The listing builds one solid part. Answer for the finished solid, in the listing's coordinates (mm). A direction names the side the tool comes from. Coordinates: 2 decimals unless noted, no trailing zeros. Loops run counter-clockwise (first coordinate to the right, second up) from the corner with the lowest first, then second, coordinate; pieces in that order, holes last. Notation, with made-up numbers: (-22.75, 76.5) - (16.25, 76.5) arc R25 cw to (16.25, 104.5) - close; hole circle Ø10 at (30.5, 14.25). An arc over 180 degrees is marked (long way). Return JSON: item names as keys, results as strings. Group by question number.
1. Find the intervals of material crossed by line 1 along Y through (x, z) = (0, 14.75); line 2 along X through (y, z) = (59, -15.5); line 3 along Y through (x, z) = (4, -17), in increasing order.
2. The mould has two halves that part along Z. Classify faces 4 (the face through (0, 59, 10)), 5 (the face through (10, 95, -15)), 6 (the face through (-1.42, 96.08, -16)): pulls with the +Z half, pulls with the -Z half, needs draft (parallel to the pull), parting line crosses it, or undercut.
3. Which of the six approach directions +Z, -Z, +X, -X, +Y, -Y give full straight-line access (tool end or side, diameter ignored) to faces 1 (the face through (-10, 95, 15)), 2 (the face through (0, 94, 12)), 3 (the face through (0, 53, -11))?
4. Section B-B (z = -13) is taken. State how many separate pieces and enclosed holes the cut face has, and give its area (3 significant figures).
5. Each of these flat-tipped pins is pushed along its axis until it touches: P1, Ø22, axis at x = -5, z = 3.5, coming from the -Y side; P2, Ø1.8, axis at x = -1.5, y = 53, coming from the +Z side; P3, Ø6, axis at y = 75.5, z = -7.5, coming from the -X side; P4, Ø10.5, axis at x = 0, y = 100, coming from the -Z side. Where does it stop, or does it pass through?
6. Section A-A (z = 0) is taken. Write down the section's boundary in (x, y).
```python
from build123d import *

# Parameters (mm, degrees)
CROQUIS1_R                 = 20
SALIENTE_EXTRUIR1_DEPTH    = 110
CORTAR_EXTRUIR1_DEPTH      = 110
CORTAR_EXTRUIR1_DEPTH_BACK = 110
CORTAR_EXTRUIR2_DEPTH      = 110
CORTAR_EXTRUIR2_DEPTH_BACK = 110
CROQUIS4_R                 = 4
CROQUIS5_R                 = 6
CORTAR_EXTRUIR4_DEPTH      = 4
CORTAR_EXTRUIR5_DEPTH      = 30
CORTAR_EXTRUIR5_DEPTH_BACK = 40
CROQUIS10_W                = 40
CROQUIS10_H                = 50
SALIENTE_EXTRUIR2_START    = 20
CROQUIS11_R                = 14
SALIENTE_EXTRUIR2_DEPTH    = 20
CROQUIS12_R                = 10
CORTAR_EXTRUIR6_DEPTH      = 18
CROQUIS14_W                = 6
CROQUIS14_H                = 2
CORTAR_EXTRUIR7_DEPTH      = 18
CROQUIS16_R                = 3
CORTAR_EXTRUIR8_DEPTH      = 9
CHAFL_N1_SIZE              = 1


with BuildPart() as part:
    # Croquis1 → Saliente-Extruir1 (new body)
    with BuildSketch(Plane(origin=(0, 0, 0), x_dir=(1, 0, 0), z_dir=(0, 1, 0))):
        with Locations(Location((0, 0, 0), (0, 0, 270))):
            Circle(CROQUIS1_R)
    extrude(amount=SALIENTE_EXTRUIR1_DEPTH)

    # Croquis2 → Cortar-Extruir1 (cut, two sides: drawn at the far end of the back side and taken through both)
    with BuildSketch(Plane.XY.offset(-CORTAR_EXTRUIR1_DEPTH_BACK)):
        with BuildLine():
            Line((-10, 90), (-10, 100))
            ThreePointArc((-10, 100), (-7.071067812, 107.071067812), (0, 110))
            Line((0, 110), (-20, 110))
            Line((-20, 110), (-20, 75.718519933))
            Line((-20, 75.718519933), (-10, 90))
        make_face()
        with BuildLine():
            Line((20, 110), (0, 110))
            ThreePointArc((0, 110), (7.071067812, 107.071067812), (10, 100))
            Line((10, 100), (10, 90))
            Line((10, 90), (20, 75.718519933))
            Line((20, 75.718519933), (20, 110))
        make_face()
    extrude(amount=CORTAR_EXTRUIR1_DEPTH + CORTAR_EXTRUIR1_DEPTH_BACK, mode=Mode.SUBTRACT)

    # Croquis4 → Cortar-Extruir2 (cut, two sides: drawn at the far end of the back side and taken through both)
    with BuildSketch(Plane.XY.offset(-CORTAR_EXTRUIR2_DEPTH_BACK)):
        with Locations(Location((0, 100, 0), (0, 0, 180))):
            Circle(CROQUIS4_R)
    extrude(amount=CORTAR_EXTRUIR2_DEPTH + CORTAR_EXTRUIR2_DEPTH_BACK, mode=Mode.SUBTRACT)

    # Croquis3 → Cortar-Revolución1 (revolve, cut)
    with BuildSketch(Plane(origin=(0, 0, 0), x_dir=(0, 0, -1), z_dir=(1, 0, 0))):
        with BuildLine():
            Line((-12, 110), (12, 110))
            Line((12, 110), (12, 84))
            ThreePointArc((12, 84), (0, 72), (-12, 84))
            Line((-12, 84), (-12, 110))
        make_face()
    revolve(axis=Axis((0, 110, 12), (0, 0, -1)), mode=Mode.SUBTRACT)

    # Croquis5 → Cortar-Extruir4 (cut)
    with BuildSketch(Plane.XY.offset(20)):
        with Locations((0, 100)):
            Circle(CROQUIS5_R)
    cortar_extruir4 = extrude(amount=-CORTAR_EXTRUIR4_DEPTH, mode=Mode.SUBTRACT)

    # Simetría1: Cortar-Extruir4 across plane
    add(cortar_extruir4.mirror(Plane.XY), mode=Mode.SUBTRACT)

    # Croquis6 → Cortar-Revolución2 (revolve, cut)
    with BuildSketch(Plane.XY, mode=Mode.PRIVATE) as cortar_revoluci_n2_sk:
        Polygon((-9, 0), (0, 0), (0, 70), (-14, 70), (-14, 30), (-9, 30), align=None)
    revolve(cortar_revoluci_n2_sk.sketch.rotate(Axis((0, 70, 0), (0, -1, 0)), 270), axis=Axis((0, 70, 0), (0, -1, 0)), mode=Mode.SUBTRACT)

    # Croquis10 → Cortar-Extruir5 (cut, two sides: drawn at the far end of the back side and taken through both)
    with BuildSketch(Plane.XY.offset(-CORTAR_EXTRUIR5_DEPTH_BACK)):
        with Locations((0, 25)):
            Rectangle(CROQUIS10_W, CROQUIS10_H)
    extrude(amount=CORTAR_EXTRUIR5_DEPTH + CORTAR_EXTRUIR5_DEPTH_BACK, mode=Mode.SUBTRACT)

    # Croquis11 → Saliente-Extruir2 (add)
    with BuildSketch(Plane.XZ.offset(-70).offset(SALIENTE_EXTRUIR2_START)):
        Circle(CROQUIS11_R)
    extrude(amount=-SALIENTE_EXTRUIR2_DEPTH)

    # Croquis12 → Cortar-Extruir6 (cut)
    with BuildSketch(Plane.XZ.offset(-50)):
        with Locations(Location((0, 0, 0), (0, 0, 270))):
            Circle(CROQUIS12_R)
    extrude(amount=-CORTAR_EXTRUIR6_DEPTH, mode=Mode.SUBTRACT)

    # Croquis14 → Cortar-Extruir7 (cut)
    with BuildSketch(Plane.XZ.offset(-50)):
        with Locations((0, -10)):
            Rectangle(CROQUIS14_W, CROQUIS14_H)
    extrude(amount=-CORTAR_EXTRUIR7_DEPTH, mode=Mode.SUBTRACT)

    # Croquis16 → Cortar-Extruir8 (cut)
    with BuildSketch(Plane(origin=(0, 0, -20), x_dir=(-1, 0, 0), z_dir=(0, 0, -1))):
        with Locations((0, 59)):
            Circle(CROQUIS16_R)
    extrude(amount=-CORTAR_EXTRUIR8_DEPTH, mode=Mode.SUBTRACT)

    # Chaflán1
    chafl_n1_edges = [part.edges().sort_by_distance(p)[0] for p in [
        (0, 50, -20),
    ]]
    chamfer(chafl_n1_edges, length=CHAFL_N1_SIZE)


solid = part.part
```
The answers:
{
 "1": {"line 1": "y = 50 to 96, 104 to 110", "line 2": "x = -12.64 to -3, 3 to 12.64", "line 3": "y = 50 to 95.53, 104.47 to 109.17"},
 "2": {"face 4": "undercut", "face 5": "needs draft", "face 6": "pulls with the -Z half"},
 "3": {"face 1": "+Z, -Z, -X, +Y", "face 2": "+Y", "face 3": "-Y"},
 "4": {"separate pieces": "1", "enclosed holes": "2", "area": "1,450 mm2"},
 "5": {"P1": "stops at y = 50", "P2": "stops at z = 19.99", "P3": "stops at x = -19.49", "P4": "stops at z = -16"},
 "6": {"outline": "(-20, 51) - (-19, 50) - (-10, 50) - (-10, 68) - (10, 68) - (10, 50) - (19, 50) - (20, 51) - (20, 75.72) - (19.03, 77.11) arc R38 cw to (-19.03, 77.11) - (-20, 75.72) - close"}
}
